Geometry: final body of the model. Coordinates: model frame, mm. Coordinates: 2 decimals unless noted, no trailing zeros. Order: outer loops, then holes, each group sorted by start corner. A loop starts at its lowest first (then second) coordinate and runs counter-clockwise, first axis right, second up. Notation, with made-up numbers: M -15,26 L 2,26 A20 cw 2,43 Z; hole C -14.75,-20.5 d4. An arc over 180 degrees is marked long. One line per question, with ' | ' between items.
from build123d import *

# Parameters (mm, degrees)
BOSS_EXTRUDE1_DEPTH = 15
SKETCH4_R           = 2
CUT_EXTRUDE1_DEPTH  = 1.3


with BuildPart() as part:
    # Sketch3 → Boss-Extrude1 (new body)
    with BuildSketch(Plane(origin=(0, 0, 0), x_dir=(0, 0, -1), z_dir=(1, 0, 0))):
        with BuildLine():
            Line((3.925, 0), (13.075, 0))
            Line((13.075, 0), (13.075, 0.3))
            Line((13.075, 0.3), (4.003802629, 0.3))
            ThreePointArc((4.003802629, 0.3), (1.921620626, 0.825652519), (-0.15, 0.259807621))
            Line((-0.15, 0.259807621), (0, 0))
            ThreePointArc((0, 0), (1.9625, 0.52585029), (3.925, 0))
        make_face()
    extrude(amount=BOSS_EXTRUDE1_DEPTH)

    # Sketch4 → Cut-Extrude1 (cut, through all)
    with BuildSketch(Plane(origin=(0, 0.3, 0), x_dir=(1, 0, 0), z_dir=(0, 1, 0))):
        with Locations((7.5, 7.075)):
            Circle(SKETCH4_R)
    extrude(amount=-CUT_EXTRUDE1_DEPTH, mode=Mode.SUBTRACT)


solid = part.part
1. Material intervals for line 1 (Z direction, x = 7.5, y = 0.15) (3 decimals); line 2 (Z direction, x = 7.5, y = 0.2) (3 decimals); line 3 (Y direction, x = 13.75, z = -7.5), sorted ascending. Write a range as [from, to].
Response values:
line 1: z = [-13.075, -9.075], [-5.075, -3.639], [-0.286, 0.087] | line 2: z = [-13.075, -9.075], [-5.075, -3.528], [-0.397, 0.115] | line 3: y = [0, 0.3]
2. Draft query along Z for faces 1 (the face through (7, 0.3, -10)), 2 (the face through (6.03, 0.15, -8.43)), 3 (the face through (7.395, 0.826, -1.952)). Return one class per face: pulls with the +Z half, pulls with the -Z half, needs draft (parallel to the pull), parting line crosses it, or undercut.
Response values:
face 1: needs draft | face 2: undercut | face 3: parting line crosses it
3. Pin query (flat end, axial travel): P1, Ø2.5, axis at x = 7, z = -8, coming from the +Y side. Return the tip coordinate at first contact, or that it passes through.
Response values:
P1: stops at y = 0.3
4. Section D-D, the plane z = -11.5. Output: boundary loops of the cut face in (x, y).
Response values:
outline: M 0,0 L 15,0 L 15,0.3 L 0,0.3 Z
5. Section B-B, the plane z = -7.5. Output: boundary loops of the cut face in (x, y).
Response values:
outline: M 0,0 L 5.55,0 L 5.55,0.3 L 0,0.3 Z; M 9.45,0 L 15,0 L 15,0.3 L 9.45,0.3 Z
